Read the model definition and answer for the solid it produces. Units are mm, in the model's axes. Face numbers are marked on the shaded views. A direction names the side the tool comes from. Coordinates: 2 decimals unless noted, no trailing zeros. Loops run counter-clockwise (first coordinate to the right, second up) from the corner with the lowest first, then second, coordinate; pieces in that order, holes last.
Q1. Section D-D (y = 5.25) is taken. Give the vertices of the cut face in (x, z).
Q2. Section A-A (x = 0) is taken. Give the vertices of the cut face in (y, z).
Q3. Straight lines are drawn through the part: line 1 (Z direction, x = -3.5, y = 3); line 2 (Z direction, x = 6.5, y = 4.75); line 3 (X direction, y = -3, z = 3.9). For each, find the intervals that lie inside material, in ascending order.
Q4. Flat-ended cylindrical pins translate along their axes: P1, Ø1, axis at x = -1.5, y = 2.5, coming from the +Z side; P2, Ø2, axis at y = 2, z = 2.5, coming from the -X side; P3, Ø1, axis at x = 6, z = 1.5, coming from the -Y side. Find the tip coordinate at first contact, or state that the pin passes through.
Q5. Which of the six approach directions +Z, -Z, +X, -X, +Y, -Y give full straight-line access (tool end or side, diameter ignored) to the marked faces 1 and 2?
Q6. The mould has two halves that part along X. Classify the marked faces 3, 4 and 5: pulls with the +X half, pulls with the -X half, needs draft (parallel to the pull), parting line crosses it, or undercut.
Q7. Section C-C (z = 1.05) is taken. Give the vertices of the cut face in (x, y).
Q8. Section B-B (y = 0) is taken. Give the vertices of the cut face in (x, z), then the cut area to 3 significant figures.
from build123d import *

# Parameters (mm, degrees)
SKETCH_1_R      = 5.7
EXTRUDE_1_DEPTH = 1.3
EXTRUDE_2_DEPTH = 2.8
EXTRUDE_3_DEPTH = 0.2


with BuildPart() as part:
    # Эскиз1 → Бобышка-Вытянуть1 (new body)
    with BuildSketch(Plane.XY):
        Circle(SKETCH_1_R)
    extrude(amount=EXTRUDE_1_DEPTH)

    # Эскиз2 → Бобышка-Вытянуть2 (add)
    with BuildSketch(Plane.XY.offset(1.3)):
        with BuildLine():
            Line((-2.5, 6.5), (2.5, 6.5))
            ThreePointArc((2.5, 6.5), (9, 0), (2.5, -6.5))
            Line((2.5, -6.5), (-2.5, -6.5))
            ThreePointArc((-2.5, -6.5), (-9, 0), (-2.5, 6.5))
        make_face()
    extrude(amount=EXTRUDE_2_DEPTH)

    # Эскиз3 → Бобышка-Вытянуть3 (add)
    with BuildSketch(Plane.XY.offset(4.1)):
        with BuildLine():
            Line((-2.5, 6.5), (2.5, 6.5))
            ThreePointArc((2.5, 6.5), (9, 0), (2.5, -6.5))
            Line((2.5, -6.5), (-2.5, -6.5))
            ThreePointArc((-2.5, -6.5), (-9, 0), (-2.5, 6.5))
        make_face()
        with BuildLine():
            Line((-2.75, 4.5), (2.75, 4.5))
            ThreePointArc((2.75, 4.5), (7.25, 0), (2.75, -4.5))
            Line((2.75, -4.5), (-2.75, -4.5))
            ThreePointArc((-2.75, -4.5), (-7.25, 0), (-2.75, 4.5))
        make_face(mode=Mode.SUBTRACT)
    extrude(amount=EXTRUDE_3_DEPTH)


solid = part.part
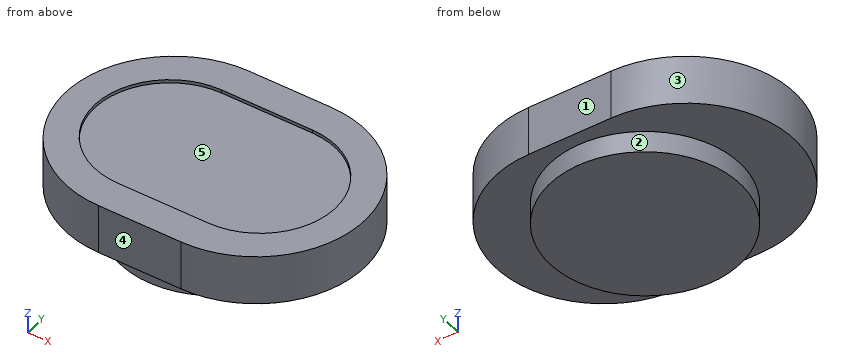
Numbers:
1. outline: (-6.33, 1.3) - (-2.22, 1.3) - (-2.22, 0) - (2.22, 0) - (2.22, 1.3) - (6.33, 1.3) - (6.33, 4.3) - (-6.33, 4.3) - close
2. outline: (-6.5, 1.3) - (-5.7, 1.3) - (-5.7, 0) - (5.7, 0) - (5.7, 1.3) - (6.5, 1.3) - (6.5, 4.3) - (4.5, 4.3) - (4.5, 4.1) - (-4.5, 4.1) - (-4.5, 4.3) - (-6.5, 4.3) - close
3. line 1: z = 0 to 4.1
3. line 2: z = 1.3 to 4.3
3. line 3: x = -8.27 to 8.27
4. P1: stops at z = 4.1
4. P2: stops at x = -8.92
4. P3: stops at y = -5.77
5. face 1: +Z, -Z, +X, -X, +Y
5. face 2: -Z
6. face 3: pulls with the -X half
6. face 4: needs draft
6. face 5: undercut
7. outline: circle Ø11.4 at (0, 0)
8. outline: (-9, 1.3) - (-5.7, 1.3) - (-5.7, 0) - (5.7, 0) - (5.7, 1.3) - (9, 1.3) - (9, 4.3) - (7.25, 4.3) - (7.25, 4.1) - (-7.25, 4.1) - (-7.25, 4.3) - (-9, 4.3) - close
8. area: 65.9 mm2
